Source: CAD feature listing. Evaluate the final solid. Frame: model axes, mm. Face numbers are marked on the shaded views. A direction names the side the tool comes from. Give positions to 0.01 mm unless a question says otherwise; leave off trailing zeros. Order: outer loops, then holes, each group sorted by start corner. A loop starts at its lowest first (then second) coordinate and runs counter-clockwise, first axis right, second up. Notation, with made-up numbers: (-16, 39) - (27, 39) arc R26 cw to (27, 56) - close; hole circle Ø11 at (16.25, 49.25). An arc over 180 degrees is marked (long way). Write each question's results on one line, items separated by ' | '. Start each with the question number.
Item 1: Section B-B on z = 0. Output: boundary loops of the cut face in (x, y), and give its area (3 significant figures).
Item 2: Section D-D on x = 43. Output: boundary loops of the cut face in (y, z), and give its area (3 significant figures).
Item 3: Line query: line 1 along Z through (x, y) = (0, -25.8); line 2 along Z through (x, y) = (0, -16.25); line 3 along X through (y, z) = (-4.25, 2). Output: solid intervals per line, ascending.
Item 4: Set-up query: the marked faces 1, 2 and 3. Return all of +Z, -Z, +X, -X, +Y, -Y with unobstructed straight access to the full face (end or side cutting, diameter ignored); none if empty.
Item 5: Contact query for flat-ended pins moving along their axis: pin 1 Ø5 at (y, z) = (-22, 51.5) entering from -X; pin 2 Ø11 at (y, z) = (-17.5, 51.5) entering from +X; pin 3 Ø11 at (x, y) = (33.5, -17.5) entering from +Z; pin 4 Ø7 at (x, z) = (0, 14.64) entering from -Y (3 decimals). Output: stop coordinate, or through.
Item 6: Section A-A on x = 0. Output: boundary loops of the cut face in (y, z), and give its area (3 significant figures).
Item 7: Section C-C on y = -26.5. Output: boundary loops of the cut face in (x, z), and give its area (3 significant figures).
```python
from build123d import *

# Parameters (mm, degrees)
F2_DEPTH = 30
F0_R     = 2.6
F0_R_2   = 6
F3_DEPTH = 50
F4_R     = 4.5
F5_DEPTH = 6
F6_W     = 30
F6_H     = 30
F7_DEPTH = 50
F8_R     = 10


with BuildPart() as f2:
    # F1 (on Front) → F2 (new body)
    with BuildSketch(Plane.XZ):
        Polygon((-50, 4.6410161514), (-50, -35.3589838486), (50, -35.3589838486), (50, 4.6410161514), (50, 24.6410161514), (50, 64.6410161514), (-50, 64.6410161514), (-50, 24.6410161514), align=None)
    extrude(amount=F2_DEPTH)

    # F0 (on Front) → F3 (cut)
    with BuildSketch(Plane.XZ):
        with Locations((0, 34.6410161514)):
            Circle(F0_R)
        with Locations((-20, 0)):
            Circle(F0_R)
        with Locations((20, 0)):
            Circle(F0_R)
        with Locations((0, 14.6410161514)):
            Circle(F0_R_2)
    extrude(amount=F3_DEPTH, mode=Mode.SUBTRACT)

    # F4 (on face) → F5 (cut)
    with BuildSketch(Plane.XZ.offset(30)):
        with Locations((0, 34.6410161514)):
            Circle(F4_R)
        with Locations((20, 0)):
            Circle(F4_R)
        with Locations((-20, 0)):
            Circle(F4_R)
    extrude(amount=-F5_DEPTH, mode=Mode.SUBTRACT)

    # F6 (on face) → F7 (cut)
    with BuildSketch(Plane(origin=(0, 0, 0), x_dir=(-1, 0, 0), z_dir=(0, 1, 0))):
        with Locations((-35, 49.6410161514)):
            Rectangle(F6_W, F6_H)
        with Locations((-35, -20.3589838486)):
            Rectangle(F6_W, F6_H)
        with Locations((35, -20.3589838486)):
            Rectangle(F6_W, F6_H)
        Polygon((50, 64.6410161514), (20.0062222363, 64.6410161514), (20.0062222363, 34.0300370508), (50, 34.6410161514), align=None)
    extrude(amount=-F7_DEPTH, mode=Mode.SUBTRACT)

    # F8
    f8_edges = [f2.edges().sort_by_distance(p)[0] for p in [
        (-20.006222, -15, 64.641016),
        (-20.006222, -15, 34.030037),
        (-50, -15, 34.641016),
        (-50, -15, -5.358984),
        (-20, -15, -5.358984),
        (-20, -15, -35.358984),
        (20, -15, -35.358984),
        (20, -15, -5.358984),
        (50, -15, -5.358984),
        (20, -15, 64.641016),
        (20, -15, 34.641016),
        (50, -15, 34.641016),
    ]]
    fillet(f8_edges, radius=F8_R)


solid = f2.part
```
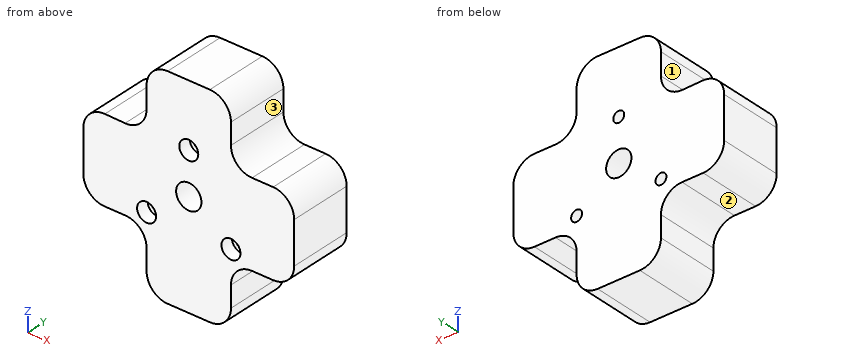
Evaluation:
1) outline: (-48.86, -30) - (-24.5, -30) - (-24.5, -24) - (-22.6, -24) - (-22.6, 0) - (-48.86, 0) - close; (-17.4, -24) - (-15.5, -24) - (-15.5, -30) - (15.5, -30) - (15.5, -24) - (17.4, -24) - (17.4, 0) - (-17.4, 0) - close; (22.6, -24) - (24.5, -24) - (24.5, -30) - (48.86, -30) - (48.86, 0) - (22.6, 0) - close | area: 2,570 mm^2
2) outline: (-30, -4.9) - (0, -4.9) - (0, 34.18) - (-30, 34.18) - close | area: 1,170 mm^2
3) line 1: z = -35.36 to 8.64, 20.64 to 30.14, 39.14 to 64.64 | line 2: z = -35.36 to 8.64, 20.64 to 32.04, 37.24 to 64.64 | line 3: x = -49.64 to -21.66, -18.34 to 18.34, 21.66 to 49.64
4) face 1: +Z, -X, +Y, -Y | face 2: -Z, -X, +Y, -Y | face 3: +Z, +X, +Y, -Y
5) pin 1: stops at x = -20.01 | pin 2: stops at x = 20 | pin 3: stops at z = 34.84 | pin 4: passes through
6) outline: (-30, -35.36) - (0, -35.36) - (0, 8.64) - (-30, 8.64) - close; (-30, 20.64) - (0, 20.64) - (0, 32.04) - (-24, 32.04) - (-24, 30.14) - (-30, 30.14) - close; (-30, 39.14) - (-24, 39.14) - (-24, 37.24) - (0, 37.24) - (0, 64.64) - (-30, 64.64) - close | area: 2,460 mm^2
7) outline: (-50, 4.64) arc R10 ccw to (-40, -5.36) - (-30, -5.36) arc R10 cw to (-20, -15.36) - (-20, -25.36) arc R10 ccw to (-10, -35.36) - (10, -35.36) arc R10 ccw to (20, -25.36) - (20, -15.36) arc R10 cw to (30, -5.36) - (40, -5.36) arc R10 ccw to (50, 4.64) - (50, 24.64) arc R10 ccw to (40, 34.64) - (30, 34.64) arc R10 cw to (20, 44.64) - (20, 54.64) arc R10 ccw to (10, 64.64) - (-10.01, 64.64) arc R10 ccw to (-20.01, 54.64) - (-20.01, 44.24) arc R10 cw to (-30.21, 34.24) - (-39.8, 34.43) arc R10 ccw to (-50, 24.44) - close; hole circle Ø9 at (-20, 0); hole circle Ø12 at (0, 14.64); hole circle Ø9 at (0, 34.64); hole circle Ø9 at (20, 0) | area: 6,000 mm^2
